Print and shaded views of the part. All mm, measured from the part's lowest x, y and z. Coordinates: 2 decimals unless noted, no trailing zeros. Loops run counter-clockwise (first coordinate to the right, second up) from the corner with the lowest first, then second, coordinate; pieces in that order, holes last. Notation, with made-up numbers: M 22,5 L 72,5 A9 ccw 72,17 Z; hole C 42,-36.75 d4. An arc over 180 degrees is marked long. Answer as a JSON object with one key per item and string values. Group by question number.
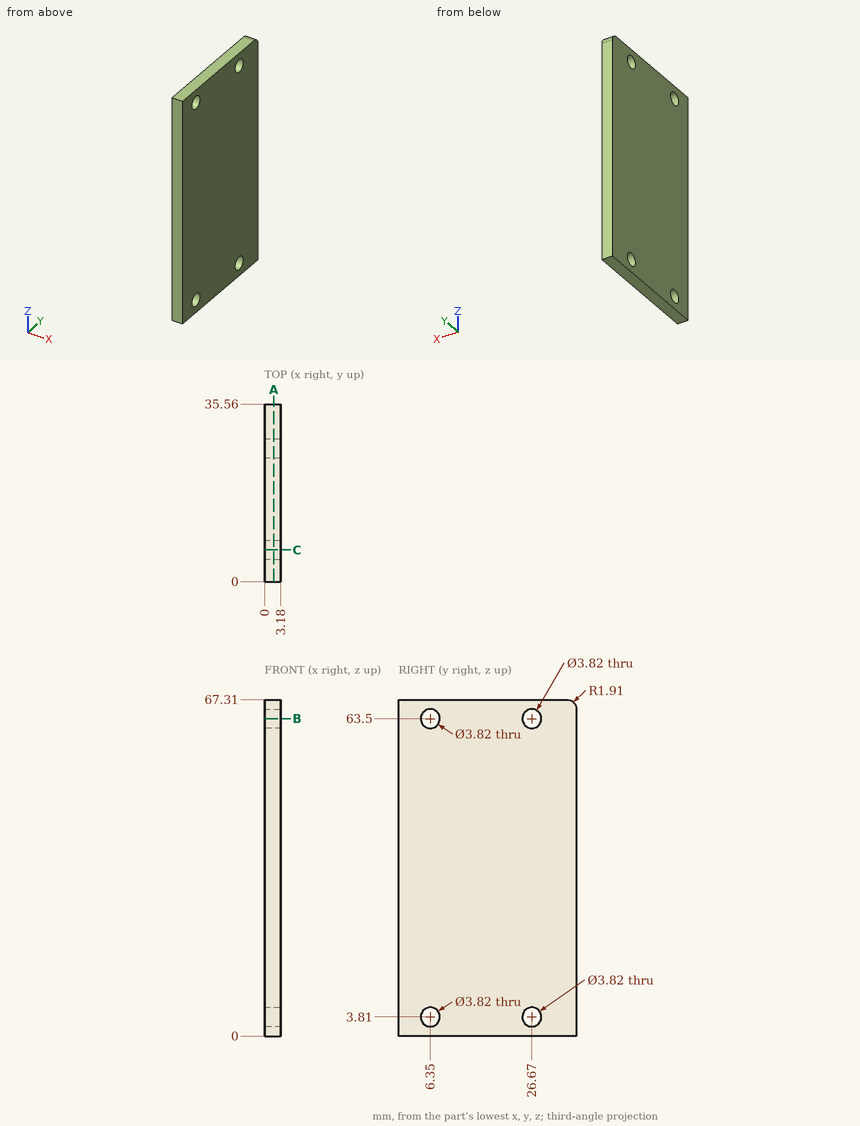
Item 1: Pin check, flat tip, straight feed: pin 1 (3.5 mm diameter, centred on y = 26.67, z = 3.81, fed in from -X). Stop position of the tip, or through.
Item 2: Slice it at A-A, the plane x = 1.85. Write the cut outline in (y, z), then the cut area to 3 significant figures.
Item 3: Slice it at C-C, the plane y = 6.35. Write the cut outline in (x, z), then the cut area to 3 significant figures.
Item 4: Slice it at B-B, the plane z = 63.5. Write the cut outline in (x, y), then the cut area to 3 significant figures.
Item 5: Drill centre lines: L1, parallel to Y at x = 1.8, z = 63.5; L2, parallel to Y at x = 2.55, z = 65. Where is each one in solid material? Low to high. Write a range as from..to.
Computed:
{
 "1": {"pin 1": "through"},
 "2": {"outline": "M 0,0 L 35.56,0 L 35.56,65.4 A1.91 ccw 33.65,67.31 L 0,67.31 Z; hole C 6.35,3.81 d3.82; hole C 6.35,63.5 d3.82; hole C 26.67,3.81 d3.82; hole C 26.67,63.5 d3.82", "area": "2,350 mm2"},
 "3": {"outline": "M 0,0 L 3.18,0 L 3.18,1.9 L 0,1.9 Z; M 0,5.72 L 3.18,5.72 L 3.18,61.59 L 0,61.59 Z; M 0,65.41 L 3.18,65.41 L 3.18,67.31 L 0,67.31 Z", "area": "190 mm2"},
 "4": {"outline": "M 0,0 L 3.18,0 L 3.18,4.44 L 0,4.44 Z; M 0,8.26 L 3.18,8.26 L 3.18,24.76 L 0,24.76 Z; M 0,28.58 L 3.18,28.58 L 3.18,35.56 L 0,35.56 Z", "area": "88.8 mm2"},
 "5": {"L1": "0..4.44, 8.26..24.76, 28.58..35.56", "L2": "0..5.17, 7.53..25.49, 27.85..35.56"}
}
